Can you work these out from the model? Positions are in its coordinate system, mm. Give positions to 0.01 mm unless a question says otherwise; leave off trailing zeros. Order: outer loops, then holes, each group sorted by start corner. A loop starts at its lowest first (then second) coordinate and runs counter-clockwise, first axis right, second up. Notation, with made-up numbers: (-26.75, 45.25) - (16.25, 45.25) arc R23 cw to (16.25, 67.25) - close; hole circle Ø1 at (-6.5, 27.5). An arc over 180 degrees is marked (long way). One line per question, with ' | ' between items.
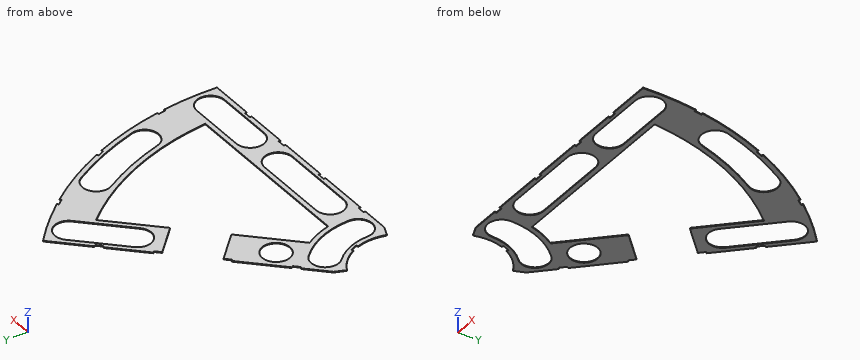
```python
from build123d import *

# Parameters (mm, degrees)
BOSS_EXTRUDE1_DEPTH = 0.254
SKETCH2_R           = 4.699
CUT_EXTRUDE1_DEPTH  = 1.254
SKETCH3_W           = 2.54
SKETCH3_H           = 0.635
CUT_EXTRUDE2_DEPTH  = 1.254
CUT_EXTRUDE4_DEPTH  = 1.254
CUT_EXTRUDE5_DEPTH  = 1.254


with BuildPart() as part:
    # Sketch1 → Boss-Extrude1 (new body)
    with BuildSketch(Plane.XY):
        with BuildLine():
            Line((67.21146711, 76.191723231), (8.696654013, 17.676910134))
            Line((8.696654013, 17.676910134), (7.228954972, 14.133571205))
            ThreePointArc((7.228954972, 14.133571205), (14.666587579, 6.075099489), (15.105587123, -4.88230096))
            Line((15.105587123, -4.88230096), (18.648926052, -6.35))
            Line((18.648926052, -6.35), (101.401368334, -6.35))
            ThreePointArc((101.401368334, -6.35), (93.866160503, 38.880636728), (67.21146711, 76.191723231))
        make_face()
        with BuildLine():
            Line((88.672924278, 6.35), (27.86051193, 6.35))
            ThreePointArc((27.86051193, 6.35), (26.399857642, 10.93517908), (24.190484974, 15.210228852))
            Line((24.190484974, 15.210228852), (67.191354125, 58.211098004))
            ThreePointArc((67.191354125, 58.211098004), (82.13289044, 34.020557137), (88.672924278, 6.35))
        make_face(mode=Mode.SUBTRACT)
    extrude(amount=BOSS_EXTRUDE1_DEPTH)

    # Sketch2 → Cut-Extrude1 (cut, through all)
    with BuildSketch(Plane.XY.offset(0.254)):
        with Locations((22.225, 0)):
            Circle(SKETCH2_R)
        with Locations((36.195, 0)):
            Circle(SKETCH2_R)
        with Locations((61.722, 0)):
            Circle(SKETCH2_R)
        with Locations((75.692, 0)):
            Circle(SKETCH2_R)
        with Locations((95.25, 0)):
            Circle(SKETCH2_R)
        with Locations((15.715448212, 15.715448212)):
            Circle(SKETCH2_R)
        with Locations((25.593729945, 25.593729945)):
            Circle(SKETCH2_R)
        with Locations((43.644044748, 43.644044748)):
            Circle(SKETCH2_R)
        with Locations((53.522326482, 53.522326482)):
            Circle(SKETCH2_R)
        with Locations((92.004434954, 24.652514046)):
            Circle(SKETCH2_R)
        with Locations((82.48891971, 47.625)):
            Circle(SKETCH2_R)
        with Locations((67.351920908, 67.351920908)):
            Circle(SKETCH2_R)
    extrude(amount=-CUT_EXTRUDE1_DEPTH, mode=Mode.SUBTRACT)

    # Sketch3 → Cut-Extrude2 (cut, through all)
    with BuildSketch(Plane.XY.offset(0.254)):
        Polygon((15.266435406, 24.246691527), (17.06248663, 26.042742751), (17.511499436, 25.593729945), (15.715448212, 23.797678721), align=None)
        Polygon((44.991083167, 53.971339288), (43.195031942, 52.175288063), (43.644044748, 51.726275257), (45.440095973, 53.522326482), align=None)
        with Locations((29.21, -6.0325)):
            Rectangle(SKETCH3_W, SKETCH3_H)
        with Locations((68.707, -6.0325)):
            Rectangle(SKETCH3_W, SKETCH3_H)
        Polygon((29.230733674, 38.210989795), (31.026784898, 40.007041019), (31.475797704, 39.558028213), (29.67974648, 37.761976989), align=None)
        Polygon((56.845021246, 65.825277367), (55.048970022, 64.029226143), (55.497982828, 63.580213337), (57.294034052, 65.376264561), align=None)
        with Locations((48.9585, -6.0325)):
            Rectangle(SKETCH3_W, SKETCH3_H)
        with Locations((85.471, -6.0325)):
            Rectangle(SKETCH3_W, SKETCH3_H)
        Polygon((99.935462164, 14.437711971), (100.266998693, 11.919442024), (101.526133667, 12.085210288), (101.194597138, 14.603480236), align=None)
        Polygon((93.765504959, 37.464305742), (94.938831965, 37.950313702), (93.966816047, 40.296967714), (92.793489041, 39.810959755), align=None)
        Polygon((79.327792988, 62.471156422), (80.874047017, 60.456038938), (81.88160576, 61.229165953), (80.33535173, 63.244283437), align=None)
        Polygon((13.593916116, 7.005422516), (14.565932035, 4.658768503), (15.739259041, 5.144776462), (14.767243123, 7.491430475), align=None)
    extrude(amount=-CUT_EXTRUDE2_DEPTH, mode=Mode.SUBTRACT)

    # Sketch6 → Cut-Extrude4 (cut, through all)
    with BuildSketch(Plane.XY.offset(0.254)):
        with BuildLine():
            Line((50.199631717, 56.845021246), (64.029226143, 70.674615673))
            ThreePointArc((64.029226143, 70.674615673), (70.674615673, 70.674615673), (70.674615673, 64.029226143))
            Line((70.674615673, 64.029226143), (56.845021246, 50.199631717))
            ThreePointArc((56.845021246, 50.199631717), (50.199631717, 50.199631717), (50.199631717, 56.845021246))
        make_face()
        with BuildLine():
            Line((61.722, -4.699), (36.195, -4.699))
            ThreePointArc((36.195, -4.699), (31.496, 0), (36.195, 4.699))
            Line((36.195, 4.699), (61.722, 4.699))
            ThreePointArc((61.722, 4.699), (66.421, 0), (61.722, -4.699))
        make_face()
        with BuildLine():
            Line((95.25, -4.699), (75.692, -4.699))
            ThreePointArc((75.692, -4.699), (70.993, 0), (75.692, 4.699))
            Line((75.692, 4.699), (95.25, 4.699))
            ThreePointArc((95.25, 4.699), (99.949, 0), (95.25, -4.699))
        make_face()
        with BuildLine():
            ThreePointArc((26.924, 0), (24.874532533, 10.303368733), (19.038142977, 19.038142977))
            ThreePointArc((19.038142977, 19.038142977), (12.392753447, 19.038142977), (12.392753447, 12.392753447))
            ThreePointArc((12.392753447, 12.392753447), (16.191912687, 6.706909836), (17.526, 0))
            ThreePointArc((17.526, 0), (22.225, -4.699), (26.924, 0))
        make_face()
        with BuildLine():
            ThreePointArc((96.543320412, 25.868704739), (92.340835395, 38.248826381), (86.558373083, 49.9745))
            ThreePointArc((86.558373083, 49.9745), (80.13941971, 51.694453372), (78.419466338, 45.2755))
            ThreePointArc((78.419466338, 45.2755), (83.658215548, 34.652367484), (87.465549496, 23.436323353))
            ThreePointArc((87.465549496, 23.436323353), (93.220625647, 20.113628588), (96.543320412, 25.868704739))
        make_face()
    extrude(amount=-CUT_EXTRUDE4_DEPTH, mode=Mode.SUBTRACT)

    # Sketch5 → Cut-Extrude5 (cut, through all)
    with BuildSketch(Plane.XY.offset(0.254)):
        Polygon((30.038956725, 40.81526407), (42.386808891, 53.163116237), (53.163116237, 42.386808891), (40.81526407, 30.038956725), align=None)
    extrude(amount=-CUT_EXTRUDE5_DEPTH, mode=Mode.SUBTRACT)


solid = part.part
```
(1) Imagine slicing it at C-C (z = 0.2). Count the separate pieces of the cut face and the enclosed holes in it, and give its area (3 significant figures).
Answer below:
separate pieces: 1 | enclosed holes: 6 | area: 1,360 mm^2
(2) Will these pins go through, and if not, where does the flat tip stop? pin 1 (2 mm diameter, centred on x = 25.5, y = 27.5, fed in from +Z); pin 2 (2 mm diameter, centred on x = 63.5, y = 7, fed in from -Z).
Answer below:
pin 1: through | pin 2: z = 0
(3) Imagine slicing it at A-A (y = 28). List the corners of the cut face in (x, z) for me.
Answer below:
outline: (19.02, 0) - (21.56, 0) - (21.56, 0.25) - (19.02, 0.25) - close; (29.63, 0) - (36.98, 0) - (36.98, 0.25) - (29.63, 0.25) - close; (84.38, 0) - (86.11, 0) - (86.11, 0.25) - (84.38, 0.25) - close; (95.95, 0) - (97.67, 0) - (97.67, 0.25) - (95.95, 0.25) - close
(4) If I drill on line 1 (Y direction, x = 57.5, z = 0.2); line 2 (Y direction, x = 81, z = 0.15); line 3 (Y direction, x = 36, z = 0.2), over which ranges is the centre line in solid material (lowest first)?
Answer below:
line 1: -6.35 to -4.7, 4.7 to 6.35, 48.52 to 50.85, 64.15 to 66.48 | line 2: -6.35 to -4.7, 4.7 to 6.35, 36.64 to 40.48, 52.08 to 60.55 | line 3: -6.35 to -4.69, 4.69 to 6.35, 27.02 to 34.85
(5) Imagine slicing it at B-B (x = 53.5). List the corners of the cut face in (y, z) for me.
Answer below:
outline: (-6.35, 0) - (-4.7, 0) - (-4.7, 0.25) - (-6.35, 0.25) - close; (4.7, 0) - (6.35, 0) - (6.35, 0.25) - (4.7, 0.25) - close; (44.52, 0) - (48.82, 0) - (48.82, 0.25) - (44.52, 0.25) - close; (60.15, 0) - (62.48, 0) - (62.48, 0.25) - (60.15, 0.25) - close
